Verification items for the finished model (mm, model axes). A direction names the side the tool comes from. Round coordinates to 2 decimals unless told otherwise and drop trailing zeros. Write each loop counter-clockwise with the first axis right and the second up, starting at its lowest first coordinate (ties: lowest second). Pieces come first, ordered by that corner, then holes.
from build123d import *

# Parameters (mm, degrees)
F1_DEPTH = 20
F2_DEPTH = 40
F3_R     = 25
F4_DEPTH = 15
F5_R     = 12.5
F6_DEPTH = 10
F8_DEPTH = 10
F9_R     = 10


with BuildPart() as f1:
    # F0 (on Top) → F1 (new body)
    with BuildSketch(Plane.XY):
        with BuildLine():
            ThreePointArc((0, 50), (35.355339, 35.355339), (50, 0))
            ThreePointArc((50, 0), (49.746808, -5.025448), (48.989795, -10))
            Line((48.989795, -10), (165, -10))
            Line((165, -10), (165, 50))
            Line((165, 50), (0, 50))
        make_face()
    extrude(amount=F1_DEPTH)

    # F0 (on Top) → F2 (join)
    with BuildSketch(Plane.XY):
        with BuildLine():
            Line((0, -10), (0, 50))
            ThreePointArc((0, 50), (-38.729833, -31.622777), (48.989795, -10))
            Line((48.989795, -10), (0, -10))
        make_face()
        with BuildLine():
            ThreePointArc((48.989795, -10), (49.746808, -5.025448), (50, 0))
            ThreePointArc((50, 0), (35.355339, 35.355339), (0, 50))
            Line((0, 50), (0, -10))
            Line((0, -10), (48.989795, -10))
        make_face()
    extrude(amount=F2_DEPTH)

    # F3 (on face) → F4 (cut)
    with BuildSketch(Plane.XY.offset(40)):
        Circle(F3_R)
    extrude(amount=-F4_DEPTH, mode=Mode.SUBTRACT)

    # F5 (on face) → F6 (cut)
    with BuildSketch(Plane.XY.offset(25)):
        Circle(F5_R)
    extrude(amount=-F6_DEPTH, mode=Mode.SUBTRACT)

    # F7 (on face) → F8 (cut)
    with BuildSketch(Plane.XY.offset(20)):
        with BuildLine():
            Line((155, 0), (155, 40))
            Line((155, 40), (44.72136, 40))
            ThreePointArc((44.72136, 40), (56.050342, 21.409325), (60, 0))
            Line((60, 0), (155, 0))
        make_face()
    extrude(amount=-F8_DEPTH, mode=Mode.SUBTRACT)

    # F9
    f9_edges = [f1.edges().sort_by_distance(p)[0] for p in [
        (165, 50, 10),
        (165, -10, 10),
        (155, 40, 15),
        (155, 0, 15),
    ]]
    fillet(f9_edges, radius=F9_R)


solid = f1.part
Q1. Sectioned sample at D-D (z = 35). Enter the section's corners in (x, y).
Recorded:
outline: (48.99, -10) arc R50 ccw to (50, 0) arc R50 ccw (long way) to start; hole circle Ø50 at (0, 0)
Q2. Release check for a two-part mould opening along X. For faces 4 (the flat face through (79, 50, 10)), 5 (the flat face through (0, 0, 15)), 6 (the flat face through (155, 20, 15)), 7 (the cylindrical face through (161.99, 47.15, 10.14)) record: released by +X, released by -X, zero draft, split by the parting line, or undercut.
Recorded:
face 4: zero draft
face 5: undercut
face 6: undercut
face 7: released by +X
Q3. Depth check by flat-ended pin: P1, Ø5, axis at y = -18.5, z = 14.5, coming from the -X side; P2, Ø6, axis at y = -29, z = 8, coming from the -X side; P3, Ø11, axis at y = 15, z = 13, coming from the -X side. Enter the tip coordinate at first touch or a pass-through.
Recorded:
P1: stops at x = -47.37
P2: stops at x = -42.71
P3: stops at x = -49.09
Q4. Material ranges on line 1 along Y through (x, z) = (0, 17.5); line 2 along Y through (x, z) = (0, 29); line 3 along Y through (x, z) = (143, 9), recorded low to high.
Recorded:
line 1: y = -50 to -12.5, 12.5 to 50
line 2: y = -50 to -25, 25 to 50
line 3: y = -10 to 50
Q5. Sectioned sample at A-A (x = 93). Enter the section's corners in (y, z).
Recorded:
outline: (-10, 0) - (50, 0) - (50, 20) - (40, 20) - (40, 10) - (0, 10) - (0, 20) - (-10, 20) - close
Q6. Sectioned sample at B-B (z = 4). Enter the section's corners in (x, y), plus the area to 3 significant figures.
Recorded:
outline: (0, 50) arc R50 ccw (long way) to (48.99, -10) - (155, -10) arc R10 ccw to (165, 0) - (165, 40) arc R10 ccw to (155, 50) - close
area: 15,300 mm2
Q7. Sectioned sample at C-C (y = 35). Enter the section's corners in (x, z).
Recorded:
outline: (-35.71, 0) - (165, 0) - (165, 20) - (153.66, 20) - (153.66, 10) - (48.73, 10) - (48.73, 20) - (35.71, 20) - (35.71, 40) - (-35.71, 40) - close
Q8. Tool access check on faces 1 (the cylindrical face through (49.74, -5.1, 29.86)), 2 (the cylindrical face through (23.846, 7.509, 32.605)), 3 (the flat face through (101, -10, 10)). Record the directions out of +Z, -Z, +X, -X, +Y, -Y that give a thin tool (end or side, any length) a straight path to the whole face; none if there is none.
Recorded:
face 1: +Z, +X, -Y
face 2: +Z
face 3: +Z, -Z, +X, -Y
